from build123d import *

# Parameters (mm, degrees)
SKETCH_W     = 100
SKETCH_H     = 100
PAD_DEPTH    = 25
SKETCH001_R  = 30
PAD001_DEPTH = 20
FILLET_R     = 9.906
FILLET001_R  = 5
THICKNESS_T  = -2


with BuildPart() as part:
    # Sketch → Pad (new body)
    with BuildSketch(Plane.XY):
        with Locations((50, 50)):
            Rectangle(SKETCH_W, SKETCH_H)
    extrude(amount=PAD_DEPTH)

    # Sketch001 (on Face6 of Pad) → Pad001 (join)
    with BuildSketch(Plane.XY.offset(25)):
        with Locations((50, 50)):
            Circle(SKETCH001_R)
    extrude(amount=PAD001_DEPTH)

    # Fillet
    fillet_edges = [part.edges().sort_by_distance(p)[0] for p in [
        (0, 0, 12.5),
        (100, 0, 12.5),
        (100, 100, 12.5),
        (0, 100, 12.5),
    ]]
    fillet(fillet_edges, radius=FILLET_R)

    # Fillet001
    fillet001_edges = [part.edges().sort_by_distance(p)[0] for p in [
        (0, 50, 25),
        (2.9014, 97.0986, 25),
        (2.9014, 2.9014, 25),
        (50, 100, 25),
        (50, 0, 25),
        (97.0986, 97.0986, 25),
        (97.0986, 2.9014, 25),
        (100, 50, 25),
        (20, 50, 25),
    ]]
    fillet(fillet001_edges, radius=FILLET001_R)

    # Thickness
    thickness_openings = [part.faces().sort_by_distance(p)[0] for p in [
        (50, 50, 0),
        (50, 50, 45),
    ]]
    offset(amount=THICKNESS_T, openings=thickness_openings, kind=Kind.INTERSECTION)


solid = part.part
Build history of the part. All positions in model axes, mm. A direction names the side the tool comes from. Give positions to 0.01 mm unless a question says otherwise; leave off trailing zeros. Order: outer loops, then holes, each group sorted by start corner. A loop starts at its lowest first (then second) coordinate and runs counter-clockwise, first axis right, second up. Notation, with made-up numbers: M 5.5,10.5 L 25.5,10.5 A22 ccw 25.5,41.5 Z; hole C 24.25,-12 d4. An arc over 180 degrees is marked long. Use one line per item in the form item = value.
Q1. Slice it at A-A, the plane x = 50. Write the cut outline in (y, z).
Conclusion:
outline = M 0,0 L 2,0 L 2,20 A3 cw 5,23 L 15,23 A7 ccw 22,30 L 22,45 L 20,45 L 20,30 A5 cw 15,25 L 5,25 A5 ccw 0,20 Z; M 78,30 A7 ccw 85,23 L 95,23 A3 cw 98,20 L 98,0 L 100,0 L 100,20 A5 ccw 95,25 L 85,25 A5 cw 80,30 L 80,45 L 78,45 Z
Q2. Pin check, flat tip, straight feed: P1, Ø2, axis at y = 15, z = 23.5, coming from the -X side. Stop position of the tip, or through.
Conclusion:
P1 = 0.67
Q3. Pull direction Y, two halves, no side cores. Call faces 1 (the flat face through (100, 49, 10)), 2 (the flat face through (49, 100, 10)), 3 (the cylindrical face through (2.86, 50.56, 22.1)): released by +Y, released by -Y, zero draft, split by the parting line, or undercut.
Conclusion:
face_1 = zero draft
face_2 = released by +Y
face_3 = undercut
Q4. Wall check: probe 1 along Y at (x, z) = (50, 42.25); probe 2 along X at (y, z) = (47.5, 10). Give the ranges that are in metal, low to high.
Conclusion:
probe_1 = 20 to 22, 78 to 80
probe_2 = 0 to 2, 98 to 100
Q5. Slice it at C-C, the plane z = 33.5. Write the cut outline in (x, y).
Conclusion:
outline = C 50,50 d60; hole C 50,50 d56
Q6. Which spindle directions (+Z, -Z, +X, -X, +Y, -Y) get a long thin tool onto all of the face, cutting with end or side? Do faces 4 (the flat face through (0, 49, 10)), 5 (the cylindrical face through (97.14, 49.44, 22.1)), 6 (the flat face through (29, 81, 25)). Say none if no direction does.
Conclusion:
face_4 = +Z, -Z, -X, +Y, -Y
face_5 = -Z
face_6 = +Z
